Check sheet for the drawn part. Datum: minimum x, y, z corner. Units: mm. A direction names the side the tool comes from. Coordinates: 2 decimals unless noted, no trailing zeros. Order: outer loops, then holes, each group sorted by start corner. A loop starts at its lowest first (then second) coordinate and runs counter-clockwise, first axis right, second up. Notation, with made-up numbers: (43.25, 35.5) - (55.25, 35.5) arc R11 ccw to (55.25, 49.5) - close; hole circle Ø5 at (81, 83). An arc over 180 degrees is marked (long way). Return JSON: item names as keys, results as strings. Group by question number.
Item 1: Tool access check on the marked faces 1 and 2. Record the directions out of +Z, -Z, +X, -X, +Y, -Y that give a thin tool (end or side, any length) a straight path to the whole face; none if there is none.
Item 2: Gauge pin test, flat ends, axial feed: pin 1 (1.6 mm diameter, centred on y = 23, z = 2, fed in from +X); pin 2 (1.6 mm diameter, centred on x = 41, z = 2, fed in from +Y); pin 3 (1.5 mm diameter, centred on y = 4, z = 1, fed in from +X). Record the tip position at first contact, or that the pin passes through.
Item 3: Scan lines: probe 1 along X at (y, z) = (2, 2.5); probe 2 along Y at (x, z) = (14, 0.8); probe 3 along Y at (x, z) = (20, 2.65). Record each from-to range of solid material in increasing order.
Item 4: Section check A-A on z = 1.8. Enter the section's corners in (x, y).
Item 5: Section check B-B on y = 7. Enter the section's corners in (x, z).
Item 6: Section check C-C on x = 4. Enter the section's corners in (y, z), then the cut area to 3 significant figures.
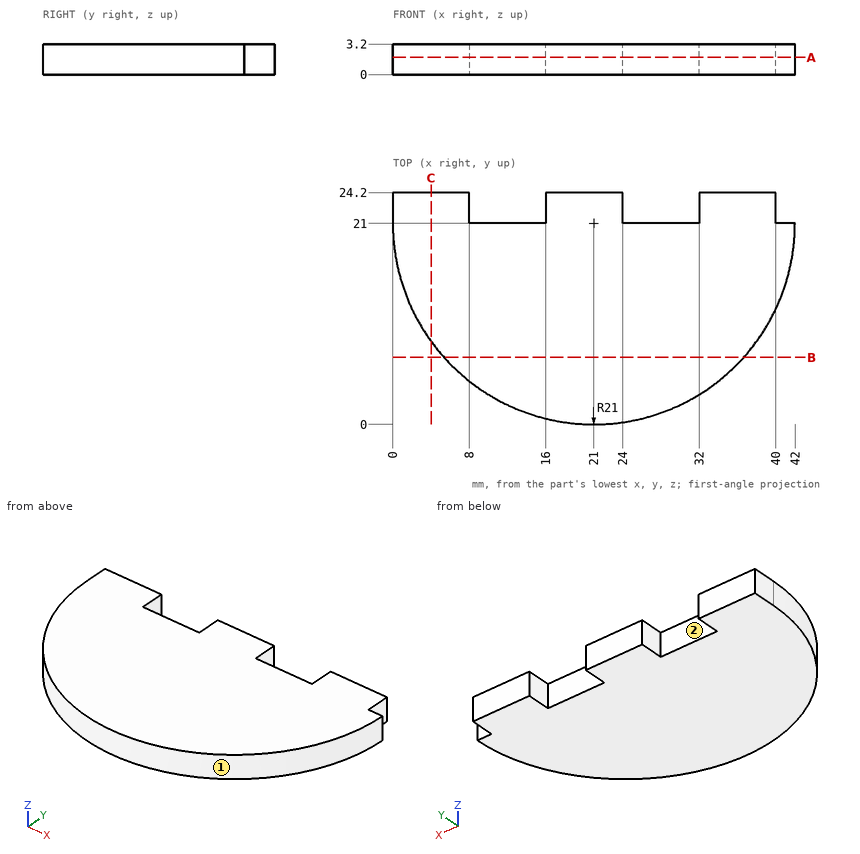
Computed:
{
 "1": {"face 1": "+Z, -Z, -Y", "face 2": "+Z, -Z, +Y"},
 "2": {"pin 1": "stops at x = 40", "pin 2": "stops at y = 21", "pin 3": "stops at x = 34.3"},
 "3": {"probe 1": "x = 12.06 to 29.94", "probe 2": "y = 1.2 to 21", "probe 3": "y = 0.02 to 24.2"},
 "4": {"outline": "(0, 21) arc R21 ccw to (42, 21) - (40, 21) - (40, 24.2) - (32, 24.2) - (32, 21) - (24, 21) - (24, 24.2) - (16, 24.2) - (16, 21) - (8, 21) - (8, 24.2) - (0, 24.2) - close"},
 "5": {"outline": "(5.35, 0) - (36.65, 0) - (36.65, 3.2) - (5.35, 3.2) - close"},
 "6": {"outline": "(8.67, 0) - (24.2, 0) - (24.2, 3.2) - (8.67, 3.2) - close", "area": "49.7 mm²"}
}
